Input: part model. Units: mm. Frame: model coordinates. A direction names the side the tool comes from. Coordinates: 2 decimals unless noted, no trailing zeros. Loops run counter-clockwise (first coordinate to the right, second up) from the corner with the lowest first, then second, coordinate; pieces in that order, holes last.
(1) Contact query for flat-ended pins moving along their axis: P1, Ø6, axis at x = 56, y = 82.62, coming from the -Z side; P2, Ø6, axis at x = 56, y = 16, coming from the +Z side; P3, Ø2.5, axis at x = 0, y = 92.62, coming from the +Z side; P4, Ø2, axis at x = -61.5, y = 92, coming from the +Z side. Output: stop coordinate, or through.
(2) Section B-B, the plane x = -56. Return loops of the section in (y, z), then the cut area to 3 significant figures.
(3) Line query: L1, parallel to X at y = 6, z = 2.35; L2, parallel to Y at x = -66.5, z = 2.7; L3, parallel to Y at x = 61.91, z = 14.1. Output: solid intervals per line, ascending.
(4) Section D-D, the plane x = -40. Return loops of the section in (y, z), then the cut area to 3 significant figures.
(5) Set-up query: faces 5 (the face through (51, 81, -4)), 6 (the face through (-62, 48, 11)), 7 (the face through (59.23, 9.79, -1.27)). Return all of +Z, -Z, +X, -X, +Y, -Y with unobstructed straight access to the full face (end or side cutting, diameter ignored); none if empty.
(6) Mould query, pull axis X, two halves, no side actions, for faces 1 (the face through (-62, 92, 11)), 2 (the face through (51.95, 12.9, -3.6)), 3 (the face through (-69.7, 49, 1)), 4 (the face through (64, 46, 17)). Classes: released by +X, released by -X, zero draft, split by the parting line, or undercut.
(7) Section A-A, the plane z = 13. Return loops of the section in (x, y) (3 decimals).
(8) Section C-C, the plane z = 5. Return loops of the section in (x, y) (3 decimals), then the cut area to 3 significant figures.
```python
from build123d import *

# Parameters (mm, degrees)
BOSS_EXTRUDE1_DEPTH                               = 3
SKETCH4_W                                         = 7
SKETCH4_H                                         = 4
SKETCH5_W                                         = 7
SKETCH5_H                                         = 4
SKETCH6_W                                         = 7
SKETCH6_H                                         = 4
SKETCH7_W                                         = 7
SKETCH7_H                                         = 4
SKETCH8_W                                         = 4
SKETCH8_H                                         = 14
SKETCH9_W                                         = 4
SKETCH9_H                                         = 14
SKETCH10_W                                        = 4
SKETCH10_H                                        = 14
SKETCH11_W                                        = 4
SKETCH11_H                                        = 14
CSK_FOR_4_FLAT_HEAD_MACHINE_SCREW_100_D           = 3.4
CSK_FOR_4_FLAT_HEAD_MACHINE_SCREW_100_DEPTH       = 17
CSK_FOR_4_FLAT_HEAD_MACHINE_SCREW_100_CSINK_D     = 6.6
CSK_FOR_4_FLAT_HEAD_MACHINE_SCREW_100_CSINK_ANGLE = 88.289805
F_6_CLEARANCE_HOLE1_D                             = 4.2
F_6_CLEARANCE_HOLE1_DEPTH                         = 6
F_3_8_CLEARANCE_HOLE1_D                           = 10.2
F_3_8_CLEARANCE_HOLE1_DEPTH                       = 0.79
FILLET1_R                                         = 1.5
FILLET2_R                                         = 2.5


with BuildPart() as part:
    # Sketch1 → Boss-Extrude1 (new body)
    with BuildSketch(Plane(origin=(0, 0, 0), x_dir=(-1, 0, 0), z_dir=(0, 0, -1))):
        with BuildLine():
            Line((-69.7, 93.82), (-69.7, 71.426225775))
            Line((-69.7, 71.426225775), (-69.7, 69.813774225))
            Line((-69.7, 69.813774225), (-69.7, 6.806225775))
            Line((-69.7, 6.806225775), (-69.7, 5.3))
            ThreePointArc((-69.7, 5.3), (-69.699314773, 5.241470835), (-69.69725947, 5.182973755))
            ThreePointArc((-69.69725947, 5.182973755), (-68.967766953, 3.532233047), (-67.317026245, 2.80274053))
            ThreePointArc((-67.317026245, 2.80274053), (-67.258529165, 2.800685227), (-67.2, 2.8))
            Line((-67.2, 2.8), (-65.693774225, 2.8))
            Line((-65.693774225, 2.8), (-0.806225775, 2.8))
            Line((-0.806225775, 2.8), (0.806225775, 2.8))
            Line((0.806225775, 2.8), (65.693774225, 2.8))
            Line((65.693774225, 2.8), (67.2, 2.8))
            ThreePointArc((67.2, 2.8), (67.258529165, 2.800685227), (67.317026245, 2.80274053))
            ThreePointArc((67.317026245, 2.80274053), (68.967766953, 3.532233047), (69.69725947, 5.182973755))
            ThreePointArc((69.69725947, 5.182973755), (69.699314773, 5.241470835), (69.7, 5.3))
            Line((69.7, 5.3), (69.7, 6.806225775))
            Line((69.7, 6.806225775), (69.7, 69.813774225))
            Line((69.7, 69.813774225), (69.7, 71.426225775))
            Line((69.7, 71.426225775), (69.7, 93.82))
            Line((69.7, 93.82), (69.7, 96.32))
            Line((69.7, 96.32), (67.2, 96.32))
            Line((67.2, 96.32), (-67.2, 96.32))
            Line((-67.2, 96.32), (-69.7, 96.32))
            Line((-69.7, 96.32), (-69.7, 93.82))
        make_face()
    extrude(amount=-BOSS_EXTRUDE1_DEPTH)

    # Sketch2 → Cut-Revolve1 (revolve, cut)
    with BuildSketch(Plane(origin=(0, 70.62, 0), x_dir=(1, 0, 0), z_dir=(0, 1, 0)), mode=Mode.PRIVATE) as cut_revolve1_sk:
        Polygon((69.800194118, 0.0002), (66.5, 0.0002), (66.5, -3), (68.2, -3), (68.2, -1.648484848), align=None)
    revolve(cut_revolve1_sk.sketch.rotate(Axis((66.5, 70.62, -0.0002), (0, 0, 1)), 14.141110809), axis=Axis((66.5, 70.62, -0.0002), (0, 0, 1)), mode=Mode.SUBTRACT)

    # Sketch3 → Cut-Revolve2 (revolve, cut)
    with BuildSketch(Plane(origin=(0, 70.62, 0), x_dir=(1, 0, 0), z_dir=(0, 1, 0)), mode=Mode.PRIVATE) as cut_revolve2_sk:
        Polygon((-63.199805882, 0.0002), (-66.5, 0.0002), (-66.5, -3), (-64.8, -3), (-64.8, -1.648484848), align=None)
    revolve(cut_revolve2_sk.sketch.rotate(Axis((-66.5, 70.62, -0.0002), (0, 0, 1)), 165.858889766), axis=Axis((-66.5, 70.62, -0.0002), (0, 0, 1)), mode=Mode.SUBTRACT)

    # Sketch4 → Revolve1 (revolve)
    with BuildSketch(Plane(origin=(0, 16, 0), x_dir=(1, 0, 0), z_dir=(0, 1, 0))):
        with Locations((-52.5, 2)):
            Rectangle(SKETCH4_W, SKETCH4_H)
    revolve(axis=Axis((-56, 16, -4.000025), (0, 0, 1)))

    # Sketch5 → Revolve2 (revolve)
    with BuildSketch(Plane(origin=(0, 16, 0), x_dir=(1, 0, 0), z_dir=(0, 1, 0))):
        with Locations((59.5, 2)):
            Rectangle(SKETCH5_W, SKETCH5_H)
    revolve(axis=Axis((56, 16, -4.000025), (0, 0, 1)))

    # Sketch6 → Revolve3 (revolve)
    with BuildSketch(Plane(origin=(0, 82.62, 0), x_dir=(1, 0, 0), z_dir=(0, 1, 0))):
        with Locations((-52.5, 2)):
            Rectangle(SKETCH6_W, SKETCH6_H)
    revolve(axis=Axis((-56, 82.62, -4.000025), (0, 0, 1)))

    # Sketch7 → Revolve4 (revolve)
    with BuildSketch(Plane(origin=(0, 82.62, 0), x_dir=(1, 0, 0), z_dir=(0, 1, 0))):
        with Locations((59.5, 2)):
            Rectangle(SKETCH7_W, SKETCH7_H)
    revolve(axis=Axis((56, 82.62, -4.000025), (0, 0, 1)))

    # Sketch8 → Revolve5 (revolve)
    with BuildSketch(Plane.XZ.offset(-92.256), mode=Mode.PRIVATE) as revolve5_sk:
        with Locations((63.91, 10)):
            Rectangle(SKETCH8_W, SKETCH8_H)
    revolve(revolve5_sk.sketch.rotate(Axis((61.91, 92.256, 17.005), (0, 0, -1)), 180), axis=Axis((61.91, 92.256, 17.005), (0, 0, -1)))

    # Sketch9 → Revolve6 (revolve)
    with BuildSketch(Plane.XZ.offset(-92.256), mode=Mode.PRIVATE) as revolve6_sk:
        with Locations((-59.915, 10)):
            Rectangle(SKETCH9_W, SKETCH9_H)
    revolve(revolve6_sk.sketch.rotate(Axis((-61.915, 92.256, 17.005), (0, 0, -1)), 180), axis=Axis((-61.915, 92.256, 17.005), (0, 0, -1)))

    # Sketch10 → Revolve7 (revolve)
    with BuildSketch(Plane.XZ.offset(-48.06), mode=Mode.PRIVATE) as revolve7_sk:
        with Locations((63.91, 10)):
            Rectangle(SKETCH10_W, SKETCH10_H)
    revolve(revolve7_sk.sketch.rotate(Axis((61.91, 48.06, 17.005), (0, 0, -1)), 180), axis=Axis((61.91, 48.06, 17.005), (0, 0, -1)))

    # Sketch11 → Revolve8 (revolve)
    with BuildSketch(Plane.XZ.offset(-48.06), mode=Mode.PRIVATE) as revolve8_sk:
        with Locations((-59.915, 10)):
            Rectangle(SKETCH11_W, SKETCH11_H)
    revolve(revolve8_sk.sketch.rotate(Axis((-61.915, 48.06, 17.005), (0, 0, -1)), 180), axis=Axis((-61.915, 48.06, 17.005), (0, 0, -1)))

    # CSK for #4 Flat Head Machine Screw (100)1
    with Locations(Plane(origin=(0, 0, 0), x_dir=(-1, 0, 0), z_dir=(0, 0, -1))):
        with Locations((66.5, 6), (0, 6), (-66.5, 6), (0, 92.62)):
            CounterSinkHole(CSK_FOR_4_FLAT_HEAD_MACHINE_SCREW_100_D / 2, CSK_FOR_4_FLAT_HEAD_MACHINE_SCREW_100_CSINK_D / 2, depth=CSK_FOR_4_FLAT_HEAD_MACHINE_SCREW_100_DEPTH, counter_sink_angle=CSK_FOR_4_FLAT_HEAD_MACHINE_SCREW_100_CSINK_ANGLE)

    # #6 Clearance Hole1
    with Locations(Plane.XY.offset(17)):
        with Locations((-61.915, 48.06), (61.91, 48.06), (-61.915, 92.256), (61.91, 92.256)):
            Hole(F_6_CLEARANCE_HOLE1_D / 2, depth=F_6_CLEARANCE_HOLE1_DEPTH)

    # 3/8 Clearance Hole1
    with Locations(Plane(origin=(0, 0, -4), x_dir=(-1, 0, 0), z_dir=(0, 0, -1))):
        with Locations((-56, 82.62), (56, 82.62), (-56, 16), (56, 16)):
            Hole(F_3_8_CLEARANCE_HOLE1_D / 2, depth=F_3_8_CLEARANCE_HOLE1_DEPTH)

    # Fillet1
    fillet1_edges = [part.edges().sort_by_distance(p)[0] for p in [
        (-63, 82.62, -4),
        (49, 82.62, -4),
        (-63, 16, -4),
        (49, 16, -4),
    ]]
    fillet(fillet1_edges, radius=FILLET1_R)

    # Fillet2
    fillet2_edges = [part.edges().sort_by_distance(p)[0] for p in [
        (69.7, 96.32, 1.5),
        (-69.7, 96.32, 1.5),
    ]]
    fillet(fillet2_edges, radius=FILLET2_R)


solid = part.part
```
Report:
1. P1: stops at z = -3.21
1. P2: stops at z = 3
1. P3: passes through
1. P4: stops at z = 11
2. outline: (2.8, 0) - (9, 0) - (9, -2.5) arc R1.5 ccw to (10.5, -4) - (10.9, -4) - (10.9, -3.21) - (21.1, -3.21) - (21.1, -4) - (21.5, -4) arc R1.5 ccw to (23, -2.5) - (23, 0) - (75.62, 0) - (75.62, -2.5) arc R1.5 ccw to (77.12, -4) - (77.52, -4) - (77.52, -3.21) - (87.72, -3.21) - (87.72, -4) - (88.12, -4) arc R1.5 ccw to (89.62, -2.5) - (89.62, 0) - (96.32, 0) - (96.32, 3) - (2.8, 3) - close
2. area: 375 mm2
3. L1: x = -69.7 to -68.2, -64.8 to -1.7, 1.7 to 64.8, 68.2 to 69.7
3. L2: y = 2.8 to 4.3, 7.7 to 68.92, 72.32 to 96.32
3. L3: y = 44.06 to 45.96, 50.16 to 52.06, 88.26 to 90.16, 94.36 to 96.26
4. outline: (2.8, 0) - (96.32, 0) - (96.32, 3) - (2.8, 3) - close
4. area: 281 mm2
5. face 5: -Z, +X, -X, +Y, -Y
5. face 6: +Z
5. face 7: -Z
6. face 1: undercut
6. face 2: undercut
6. face 3: released by -X
6. face 4: zero draft
7. outline: circle Ø8 at (-61.915, 48.06); circle Ø8 at (-61.915, 92.256); circle Ø8 at (61.91, 48.06); circle Ø8 at (61.91, 92.256); hole circle Ø4.2 at (-61.915, 48.06); hole circle Ø4.2 at (-61.915, 92.256); hole circle Ø4.2 at (61.91, 48.06); hole circle Ø4.2 at (61.91, 92.256)
8. outline: circle Ø8 at (-61.915, 48.06); circle Ø8 at (-61.915, 92.256); circle Ø8 at (61.91, 48.06); circle Ø8 at (61.91, 92.256)
8. area: 201 mm2
